Source: CAD feature listing. Evaluate the final solid. Frame: model axes, mm. Give positions to 0.01 mm unless a question says otherwise; leave off trailing zeros. Loops run counter-clockwise (first coordinate to the right, second up) from the corner with the lowest first, then second, coordinate; pieces in that order, holes last. Notation, with made-up numbers: (-23, -11.75) - (-2, -11.75) arc R9 ccw to (-2, -2.75) - close; hole circle Ø6 at (-5.75, -4.75). An arc over 180 degrees is marked (long way). Put each result on its own line as item: value.
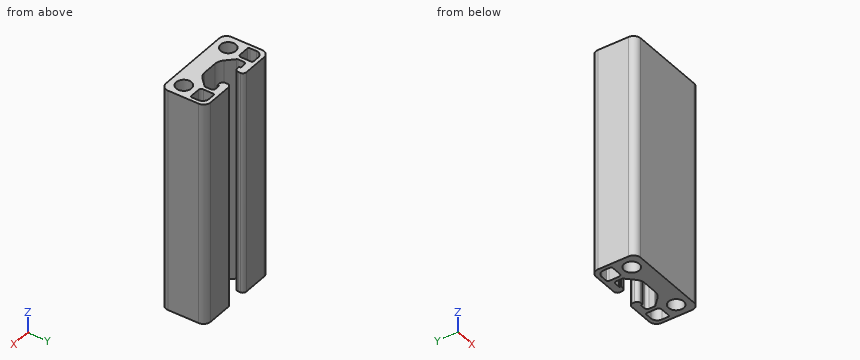
Autodesk Inventor part; units mm, degrees
ref_plane "YZ Plane" through (0, 0, 0) normal (1, 0, 0) x (0, 1, 0)
ref_plane "XZ Plane" through (0, 0, 0) normal (0, 1, 0) x (-1, 0, 0)
ref_plane "XY Plane" through (0, 0, 0) normal (0, 0, 1) x (1, 0, 0)
sketch "Sketch1" plane through (0, 0, 0) normal (0, 0, 1) x (1, 0, 0)
  arc A0 (17.687, 1.9459) -> (18.324, 2.5123) centre (17.6928, 2.5809) ccw
  line L0 (13.2104, 1.9459) -> (17.687, 1.9459)
  arc A1 (11.9404, 3.2159) -> (13.2104, 1.9459) centre (13.2104, 3.2159) ccw
  line L1 (11.9404, 7.6925) -> (11.9404, 3.2159)
  arc A2 (12.5686, 8.3275) -> (11.9404, 7.6925) centre (12.5754, 7.6925) ccw
  line L2 (15.5601, 8.3275) -> (12.5686, 8.3275)
  arc A3 (18.324, 5.5037) -> (15.5601, 8.3275) centre (15.5302, 5.5336) ccw
  line L3 (18.324, 2.5123) -> (18.324, 5.5037)
  circle A4 centre (14, -4) radius 3.4036
  circle A5 centre (-14, -4) radius 3.4036
  arc A6 (-13.2123, 1.9392) -> (-11.9423, 3.2092) centre (-13.2123, 3.2092) ccw
  line L4 (-17.6889, 1.9392) -> (-13.2123, 1.9392)
  arc A7 (-18.3171, 2.5742) -> (-17.6889, 1.9392) centre (-17.6821, 2.5742) ccw
  line L5 (-18.3171, 5.5656) -> (-18.3171, 2.5742)
  arc A8 (-15.4934, 8.3296) -> (-18.3171, 5.5656) centre (-15.5233, 5.5357) ccw
  line L6 (-12.5019, 8.3296) -> (-15.4934, 8.3296)
  arc A9 (-11.9423, 7.6857) -> (-12.5019, 8.3296) centre (-12.5772, 7.6991) ccw
  line L7 (-11.9423, 3.2092) -> (-11.9423, 7.6857)
  arc A10 (-16.825, 10) -> (-20, 6.825) centre (-16.825, 6.825) ccw
  line L8 (-20, 6.825) -> (-20, -6.825)
  arc A11 (-20, -6.825) -> (-16.825, -10) centre (-16.825, -6.825) ccw
  line L9 (-16.825, -10) -> (16.825, -10)
  arc A12 (16.825, -10) -> (20, -6.825) centre (16.825, -6.825) ccw
  line L10 (20, -6.825) -> (20, 6.825)
  arc A13 (20, 6.825) -> (16.825, 10) centre (16.825, 6.825) ccw
  line L11 (16.825, 10) -> (5.6244, 10)
  arc A14 (5.6244, 10) -> (4.06, 8.4356) centre (5.6244, 8.4356) ccw
  line L12 (4.06, 8.4356) -> (4.06, 7.5148)
  arc A15 (4.06, 7.5148) -> (5.6348, 5.94) centre (5.6348, 7.5148) ccw
  line L13 (5.6348, 5.94) -> (6.7718, 5.94)
  line L14 (6.7718, 5.94) -> (6.7718, 6.7089)
  line L15 (6.7718, 6.7089) -> (9.0158, 6.7089)
  arc A16 (10.285, 5.3946) -> (9.0158, 6.7089) centre (9.0158, 5.4389) ccw
  line L16 (10.285, 5.3946) -> (10.285, 3.0962)
  arc A17 (10.1069, 2.5504) -> (10.285, 3.0962) centre (9.3961, 3.0842) ccw
  line L17 (10.1069, 2.5504) -> (6.7378, -0.8187)
  arc A18 (3.3792, -2.3) -> (6.7378, -0.8187) centre (3.2907, 2.449) ccw
  line L18 (3.3792, -2.3) -> (-3.3792, -2.3)
  arc A19 (-6.7378, -0.8187) -> (-3.3792, -2.3) centre (-3.2907, 2.449) ccw
  line L19 (-6.7378, -0.8187) -> (-10.0246, 2.4681)
  arc A20 (-10.285, 3.0967) -> (-10.0246, 2.4681) centre (-9.396, 3.0967) ccw
  line L20 (-10.285, 3.0967) -> (-10.285, 5.3946)
  arc A21 (-9.0158, 6.7089) -> (-10.285, 5.3946) centre (-9.0158, 5.4389) ccw
  line L21 (-9.0158, 6.7089) -> (-6.7718, 6.7089)
  line L22 (-6.7718, 6.7089) -> (-6.7718, 5.94)
  line L23 (-6.7718, 5.94) -> (-5.6348, 5.94)
  arc A22 (-5.6348, 5.94) -> (-4.06, 7.5148) centre (-5.6348, 7.5148) ccw
  line L24 (-4.06, 7.5148) -> (-4.06, 8.4356)
  arc A23 (-4.06, 8.4356) -> (-5.6244, 10) centre (-5.6244, 8.4356) ccw
  line L25 (-5.6244, 10) -> (-16.825, 10)
  point P0 (0, 0)
extrude "Extrusion1" add sketch "Sketch1" against normal blind 100
properties part number "40-4020-BLACK-FB"
1) Section query A-A, the plane y = -4. Output: boundary loops of the cut face in (x, z).
Check result:
outline: (-20, -100) - (-17.4, -100) - (-17.4, 0) - (-20, 0) - close; (-10.6, -100) - (10.6, -100) - (10.6, 0) - (-10.6, 0) - close; (17.4, -100) - (20, -100) - (20, 0) - (17.4, 0) - close
2) Section query C-C, the plane x = 0. Output: boundary loops of the cut face in (y, z).
Check result:
outline: (-10, -100) - (-2.3, -100) - (-2.3, 0) - (-10, 0) - close
3) Material intervals for line 1 along Y through (x, z) = (-14, -75.5); line 2 along X through (y, z) = (6.75, -57.5); line 3 along X through (y, z) = (-3.25, -93.5), sorted ascending. Write a range as [from, to].
Check result:
line 1: [-10, -7.4], [-0.6, 1.94], [8.33, 10]
line 2: [-20, -18.04], [-11.94, -4.26], [4.26, 11.94], [18.05, 20]
line 3: [-20, -17.32], [-10.68, 10.68], [17.32, 20]
4) Pin query (flat end, axial travel): P1, Ø0.7, axis at y = 7.5, z = -26.5, coming from the -X side; P2, Ø0.5, axis at y = 8, z = -70.5, coming from the +X side; P3, Ø5, axis at x = -1.5, z = -30.5, coming from the +Y side. Return the tip coordinate at first contact, or that it passes through.
Check result:
P1: x = -19.98
P2: x = 19.86
P3: y = -2.25
5) Section query B-B, the plane z = -17. State how many separate pieces and enclosed holes the cut face has, plus the area to 3 significant figures.
Check result:
separate pieces: 1
enclosed holes: 4
area: 458 mm²
